The model under review builds one solid part; all positions refer to its coordinate system, in mm. A direction names the side the tool comes from. Give positions to 0.01 mm unless a question says otherwise; leave off trailing zeros. Order: outer loops, then holes, each group sorted by start corner. A loop starts at its lowest first (then second) coordinate and runs counter-clockwise, first axis right, second up.
```python
from build123d import *

# Parameters (mm, degrees)
PATTERN_CIRCULAR_1_COUNT = 6
CHAMFER_1_SIZE           = 0.3


with BuildPart() as part:
    # 草图1 → 旋转1 (revolve)
    with BuildSketch(Plane(origin=(0, 0, 0), x_dir=(1, 0, 0), z_dir=(0, 1, 0)), mode=Mode.PRIVATE) as revolve_1_sk:
        Polygon((27.5, 0), (33, 0), (33, -8), (29, -8), (29, -1.1), (27.5, -1.1), align=None)
    revolve(revolve_1_sk.sketch.rotate(Axis((0, 0, 0), (0, 0, 1)), 180), axis=Axis((0, 0, 0), (0, 0, 1)))

    # 草图3 → M3 螺纹孔1 (revolve, cut)
    with BuildSketch(Plane(origin=(0, 31, 8), x_dir=(0, -1, 0), z_dir=(1, 0, 0))):
        Polygon((0, 0), (0, 8), (1.525, 8), (1.25, 7.725), (1.25, 0.275), (1.525, 0), align=None)
    hole_wizard_m3_1 = revolve(axis=Axis((0, 31, 14.35), (0, 0, -1)), mode=Mode.SUBTRACT)

    # 阵列(圆周)1: M3 螺纹孔1 ×6 about axis
    pattern_circular_1_axis = Axis((0, 0, 0), (0, 0, 1))
    for i in range(1, PATTERN_CIRCULAR_1_COUNT):
        add(hole_wizard_m3_1.rotate(pattern_circular_1_axis, i * 360 / PATTERN_CIRCULAR_1_COUNT), mode=Mode.SUBTRACT)

    # 倒角1
    chamfer_1_edges = [part.edges().sort_by_distance(p)[0] for p in [
        (27.5, 0, 1.1),
        (29, 0, 8),
        (33, 0, 8),
        (33, 0, 0),
        (27.5, 0, 0),
    ]]
    chamfer(chamfer_1_edges, length=CHAMFER_1_SIZE)


solid = part.part
```
Item 1: Clearance check with flat-ended pins moving along their axes: pin 1 Ø2 at (y, z) = (13.5, 6.5) entering from -X; pin 2 Ø3 at (x, z) = (13.5, 3.5) entering from -Y; pin 3 Ø1 at (x, y) = (-20.5, -20) entering from +Z. State where each tip first meets the part, or that it passes through.
Values found:
pin 1: stops at x = -30.54
pin 2: stops at y = -30.74
pin 3: stops at z = 7.84
Item 2: Draft analysis for pull direction X (two halves, no side actions). For faces 1 (the cylindrical face through (-0.479, -29.845, 4.052)), 2 (the cylindrical face through (-13.38, 25.73, 4.35)), 3 (the flat face through (22, -20, 8)), state which applies: released by +X, released by -X, zero draft, split by the parting line, or undercut.
Values found:
face 1: undercut
face 2: undercut
face 3: zero draft
Item 3: Take a section at C-C (z = 3.75). Give the boundary of the cut face in (x, y) (3 decimals), and give its area (3 significant figures).
Values found:
outline: circle Ø66 at (0, 0); hole circle Ø58 at (0, 0); hole circle Ø2.5 at (-26.847, -15.5); hole circle Ø2.5 at (-26.847, 15.5); hole circle Ø2.5 at (0, -31); hole circle Ø2.5 at (0, 31); hole circle Ø2.5 at (26.847, -15.5); hole circle Ø2.5 at (26.847, 15.5)
area: 750 mm2
Item 4: Take a section at B-B (x = 0). Give the number of separate pieces and of enclosed holes in the cut face, and give its area (3 significant figures).
Values found:
separate pieces: 4
enclosed holes: 0
area: 26.5 mm2
Item 5: For faces 4 (the flat face through (-2, 28, 1.1)), 5 (the cylindrical face through (28.067, -15.229, 4.052)), list the 3-axis set-ups (+Z, -Z, +X, -X, +Y, -Y) from which the entire face can be reached by the end or side of a thin tool; tool diameter is ignored.
Values found:
face 4: +Z
face 5: +Z, -Z
Item 6: Take a section at A-A (y = 0). Give the boundary of the cut face in (x, z), and give its area (4 significant figures).
Values found:
outline: (-33, 0.3) - (-32.7, 0) - (-27.8, 0) - (-27.5, 0.3) - (-27.5, 0.8) - (-27.8, 1.1) - (-29, 1.1) - (-29, 7.7) - (-29.3, 8) - (-32.7, 8) - (-33, 7.7) - close; (27.5, 0.3) - (27.8, 0) - (32.7, 0) - (33, 0.3) - (33, 7.7) - (32.7, 8) - (29.3, 8) - (29, 7.7) - (29, 1.1) - (27.8, 1.1) - (27.5, 0.8) - close
area: 66.85 mm2
Item 7: For line 1 (X direction, y = -15.5, z = 2); line 2 (Y direction, x = 0.5, z = 3.25); line 3 (X direction, y = -15, z = 1), list the stretches that pass through material, from the lowest coordinate up.
Values found:
line 1: x = -29.13 to -28.1, -25.6 to -24.51, 24.51 to 25.6, 28.1 to 29.13
line 2: y = -33 to -32.15, -29.85 to -29, 29 to 29.85, 32.15 to 33
line 3: x = -29.39 to -27.99, -25.7 to -23.29, 23.29 to 25.7, 27.99 to 29.39
